from build123d import *

# Parameters (mm, degrees)
SKETCH_1_R      = 1.65
EXTRUDE_1_DEPTH = 5
EXTRUDE_2_DEPTH = 50


with BuildPart() as part:
    # 스케치1 → 보스-돌출1 (new body)
    with BuildSketch(Plane.XY):
        with BuildLine():
            Line((-25, -50), (25, -50))
            Line((25, -50), (45, 0))
            Line((45, 0), (45, 60))
            Line((45, 60), (30, 60))
            Line((30, 60), (30, 0))
            ThreePointArc((30, 0), (0, -30), (-30, 0))
            Line((-30, 0), (-30, 60))
            Line((-30, 60), (-45, 60))
            Line((-45, 60), (-45, 0))
            Line((-45, 0), (-25, -50))
        make_face()
        with Locations((-37.5, 50)):
            Circle(SKETCH_1_R, mode=Mode.SUBTRACT)
        with Locations(Location((37.5, 50, 0), (0, 0, 180))):
            Circle(SKETCH_1_R, mode=Mode.SUBTRACT)
    extrude(amount=EXTRUDE_1_DEPTH)

    # 스케치4 → 보스-돌출2 (add)
    with BuildSketch(Plane(origin=(0, 0, 0), x_dir=(-1, 0, 0), z_dir=(0, 0, -1))):
        with BuildLine():
            Line((-31.916553531, -25.840797377), (-34.284766909, -26.788082728))
            ThreePointArc((-34.284766909, -26.788082728), (0, -50), (34.284766909, -26.788082728))
            Line((34.284766909, -26.788082728), (31.916553531, -25.840797377))
            ThreePointArc((31.916553531, -25.840797377), (0, -47.449356133), (-31.916553531, -25.840797377))
        make_face()
    extrude(amount=EXTRUDE_2_DEPTH)


solid = part.part
The model under review builds one solid part; all positions refer to its coordinate system, in mm. A direction names the side the tool comes from. Round coordinates to 2 decimals unless told otherwise and drop trailing zeros. Loops run counter-clockwise (first coordinate to the right, second up) from the corner with the lowest first, then second, coordinate; pieces in that order, holes last. Notation, with made-up numbers: (14.25, 70.5) -> (25.25, 70.5) arc R32 ccw to (25.25, 101.5) -> close; hole circle Ø4 at (-24, -33). An arc over 180 degrees is marked (long way). Return JSON: item names as keys, results as strings.
(1) For line 1 (Z direction, x = 39.5, y = -8); line 2 (Y direction, x = 30, z = -14.5); line 3 (Y direction, x = -27.5, z = -32), list the stretches that pass through material, from the lowest coordinate up.
Solved:
{"line 1": "0 to 5", "line 2": "-34.6 to -29.86", "line 3": "-37.72 to -33.7"}
(2) The part is to be moulded in two halves that separate along X. For faces 1 (the flat face through (-35, -25, 2)), 2 (the cylindrical face through (-38.716, 51.115, 2.465)), 3 (the flat face through (35, -25, 2)), say which applies: released by +X, released by -X, zero draft, split by the parting line, or undercut.
Solved:
{"face 1": "released by -X", "face 2": "undercut", "face 3": "released by +X"}
(3) For pin 1 (4.5 mm diameter, centred on x = -37.5, y = 50, fed in from -Z); pin 2 (5 mm diameter, centred on x = 5, z = -32.5, fed in from -Y); pin 3 (10 mm diameter, centred on x = 15, z = -18, fed in from +Y), all flat-tipped, find the tip position at first contact; note any pin that passes through.
Solved:
{"pin 1": "z = 0", "pin 2": "y = -49.92", "pin 3": "y = -41.03"}
(4) Add section D-D on x = -17. Write out the cut boundary in (y, z).
Solved:
{"outline": "(-50, 0) -> (-45.85, 0) -> (-45.85, -50) -> (-42.95, -50) -> (-42.95, 0) -> (-24.72, 0) -> (-24.72, 5) -> (-50, 5) -> close"}
(5) Add section A-A on y = 26.5. Write out the cut boundary in (x, z), plus the area to 3 significant figures.
Solved:
{"outline": "(-45, 0) -> (-30, 0) -> (-30, 5) -> (-45, 5) -> close; (30, 0) -> (45, 0) -> (45, 5) -> (30, 5) -> close", "area": "150 mm2"}
(6) Add section C-C on y = 50. Write out the cut boundary in (x, z).
Solved:
{"outline": "(-45, 0) -> (-39.15, 0) -> (-39.15, 5) -> (-45, 5) -> close; (-35.85, 0) -> (-30, 0) -> (-30, 5) -> (-35.85, 5) -> close; (30, 0) -> (35.85, 0) -> (35.85, 5) -> (30, 5) -> close; (39.15, 0) -> (45, 0) -> (45, 5) -> (39.15, 5) -> close"}
(7) For faces 4 (the flat face through (33.084, -26.308, -24.65)), 5 (the flat face through (-33.117, -26.321, -24.65)), 6 (the cylindrical face through (-0.573, -47.445, -24.65)), list the 3-axis set-ups (+Z, -Z, +X, -X, +Y, -Y) from which the entire face can be reached by the end or side of a thin tool; tool diameter is ignored.
Solved:
{"face 4": "-Z, +X, +Y", "face 5": "-Z, -X, +Y", "face 6": "-Z, +Y"}
(8) Add section B-B on x = 37.5. Write out the cut boundary in (y, z), plus the area to 3 significant figures.
Solved:
{"outline": "(-18.75, 0) -> (48.35, 0) -> (48.35, 5) -> (-18.75, 5) -> close; (51.65, 0) -> (60, 0) -> (60, 5) -> (51.65, 5) -> close", "area": "377 mm2"}
